Could you check a few things on this model? Use its own coordinates, in mm. Face numbers are marked on the shaded views. A direction names the side the tool comes from. Coordinates: 2 decimals unless noted, no trailing zeros. Write each loop counter-clockwise with the first axis right and the second up, starting at its lowest first coordinate (ties: lowest second). Pieces come first, ordered by that corner, then holes. Notation, with made-up numbers: (82, -7) - (128, -7) arc R8 ccw to (128, 1) - close; hole circle Ø3 at (41, 69.25). An arc over 180 degrees is marked (long way). Answer as a JSON object with one key per item and string values. Group by question number.
1) On a 3-axis mill with a long thin cutter (end or side, diameter ignored), from which of +Z, -Z, +X, -X, +Y, -Y can I reach the whole of each face in a straight line? I mean the marked faces 1 and 2. Say none if no direction works.
2) If we section it at C-C (z = 57.5): Write out the boundary of the cut face in (x, y).
3) Please list where these lines run through material, in increasing order: line 1 along Z through (x, y) = (0, -53); line 2 along Y through (x, z) = (78, -83); line 3 along X through (y, z) = (-52.5, -102.5).
4) If we section it at B-B (y = 69): Write out the boundary of the cut face in (x, z).
5) If we section it at A-A (x = 39): Write out the boundary of the cut face in (y, z).
6) If we section it at D-D (x = 66): Write out the boundary of the cut face in (y, z), plus the area to 3 significant figures.
7) We'd pull the mould along X, two halves only. Please class the marked faces 3, 4 and 5: released by +X, released by -X, zero draft, split by the parting line, or undercut.
8) Will these pins go through, and if not, where does the flat tip stop? pin 1 Ø1.5 at (x, z) = (2.5, 62) entering from +Y; pin 2 Ø12 at (x, y) = (-12, -18.5) entering from -Z; pin 3 Ø8 at (x, z) = (30.5, 181.5) entering from +Y.
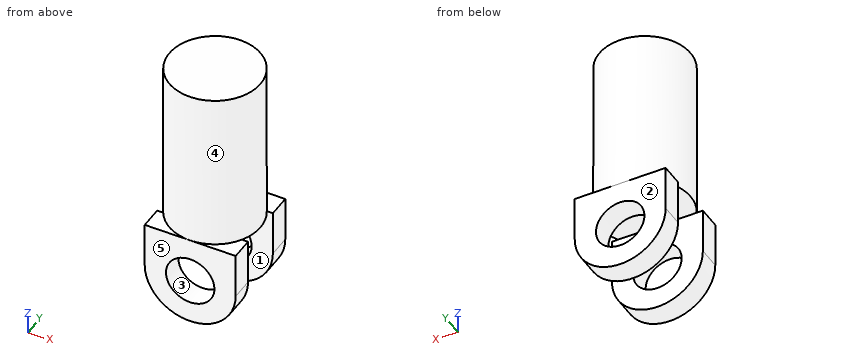
```python
from build123d import *

# Parameters (mm, degrees)
SKETCH1_R                = 90
BOSS_EXTRUDE1_DEPTH      = 320
BOSS_EXTRUDE2_DEPTH      = 90
BOSS_EXTRUDE2_DEPTH_BACK = 90
SKETCH2_R                = 48
SKETCH3_W                = 213.4354408
SKETCH3_H                = 90
CUT_EXTRUDE1_DEPTH       = 663


with BuildPart() as part:
    # Sketch1 → Boss-Extrude1 (new body)
    with BuildSketch(Plane.XY):
        Circle(SKETCH1_R)
    extrude(amount=BOSS_EXTRUDE1_DEPTH)

    # Sketch2 → Boss-Extrude2 (add, two sides: drawn at the far end of the back side and taken through both)
    with BuildSketch(Plane(origin=(0, 0, 0), x_dir=(1, 0, 0), z_dir=(0, 1, 0)).offset(-BOSS_EXTRUDE2_DEPTH_BACK)):
        with BuildLine():
            Line((90, 0), (90, 90))
            ThreePointArc((90, 90), (0, 180), (-90, 90))
            Line((-90, 90), (-90, 0))
            Line((-90, 0), (0, 0))
            Line((0, 0), (90, 0))
        make_face()
        with Locations(Location((0, 90, 0), (0, 0, 270))):
            Circle(SKETCH2_R, mode=Mode.SUBTRACT)
    extrude(amount=BOSS_EXTRUDE2_DEPTH + BOSS_EXTRUDE2_DEPTH_BACK)

    # Sketch3 → Cut-Extrude1 (cut)
    with BuildSketch(Plane.ZY.offset(90)):
        with Locations((-106.7177204, 0)):
            Rectangle(SKETCH3_W, SKETCH3_H)
    extrude(amount=-CUT_EXTRUDE1_DEPTH, mode=Mode.SUBTRACT)


solid = part.part
```
Here are the results:
{
 "1": {"face 1": "-Z, +X, -X", "face 2": "+Z, -Z, +X, -X, +Y"},
 "2": {"outline": "circle Ø180 at (0, 0)"},
 "3": {"line 1": "z = -180 to -138, -42 to 320", "line 2": "y = -90 to -45, 45 to 90", "line 3": "x = -89.13 to -46.34, 46.34 to 89.13"},
 "4": {"outline": "(-90, -90) arc R90 ccw to (90, -90) - (90, 0) - (57.78, 0) - (57.78, 320) - (-57.78, 320) - (-57.78, 0) - (-90, 0) - close; hole circle Ø96 at (0, -90)"},
 "5": {"outline": "(-90, -171.11) - (-45, -171.11) - (-45, -117.98) - (-90, -117.98) - close; (-90, -62.02) - (-45, -62.02) - (-45, 0) - (45, 0) - (45, -62.02) - (90, -62.02) - (90, 0) - (81.11, 0) - (81.11, 320) - (-81.11, 320) - (-81.11, 0) - (-90, 0) - close; (45, -171.11) - (90, -171.11) - (90, -117.98) - (45, -117.98) - close"},
 "6": {"outline": "(-90, -151.19) - (-45, -151.19) - (-45, 0) - (45, 0) - (45, -151.19) - (90, -151.19) - (90, 0) - (61.19, 0) - (61.19, 320) - (-61.19, 320) - (-61.19, 0) - (-90, 0) - close", "area": "52,800 mm²"},
 "7": {"face 3": "undercut", "face 4": "split by the parting line", "face 5": "zero draft"},
 "8": {"pin 1": "stops at y = 89.98", "pin 2": "stops at z = 0", "pin 3": "stops at y = 86.01"}
}
